Geometry check sheet. Reference: drawing and pictorial views, mm from the part's lowest x, y, z. A direction names the side the tool comes from. Give positions to 0.01 mm unless a question says otherwise; leave off trailing zeros. Write each loop counter-clockwise with the first axis right and the second up, starting at its lowest first coordinate (ties: lowest second). Pieces come first, ordered by that corner, then holes.
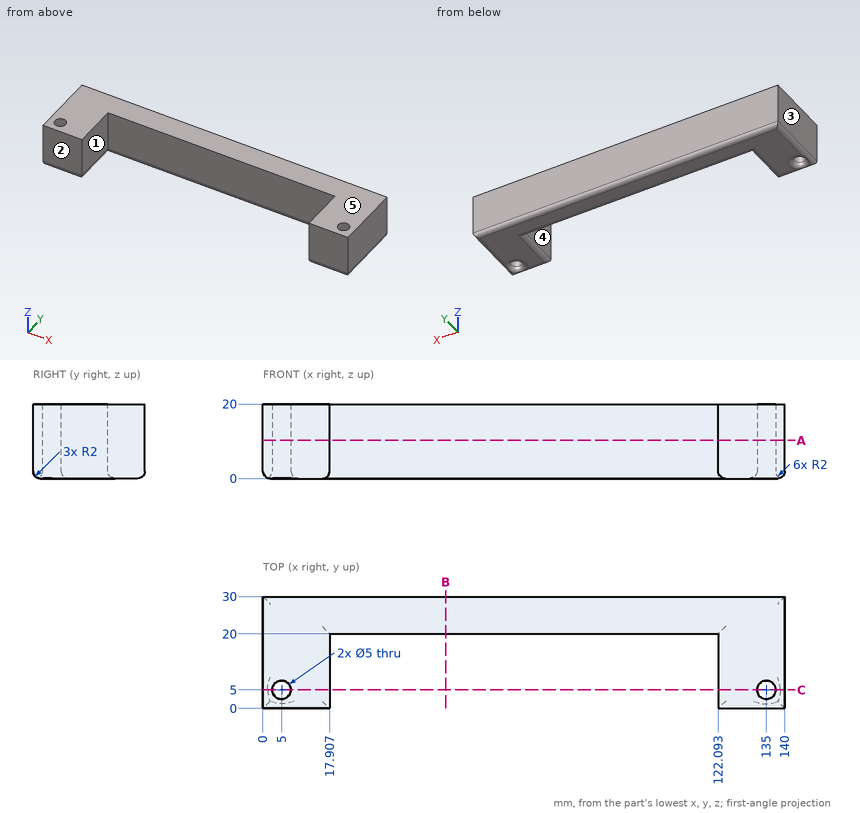
Item 1: Set-up check for the marked faces 1 and 2: record each of +Z, -Z, +X, -X, +Y, -Y from which the full face is reachable in a straight line by a thin tool's end or side.
Answer key:
face 1: +Z, -Z, -Y
face 2: +Z, -Z, +X, -X, -Y
Item 2: Depth check by flat-ended pin: pin 1 (6.5 mm diameter, centred on x = 5, y = 5, fed in from -Z); pin 2 (1 mm diameter, centred on x = 71, z = 17, fed in from -Y). Enter the tip coordinate at first touch or a pass-through.
Answer key:
pin 1: stops at z = 0.44
pin 2: stops at y = 20
Item 3: Sectioned sample at A-A on z = 10.25. Record the cut outline in (x, y), then the cut area to 3 significant figures.
Answer key:
outline: (0, 0) - (17.91, 0) - (17.91, 20) - (122.09, 20) - (122.09, 0) - (140, 0) - (140, 30) - (0, 30) - close; hole circle Ø5 at (5, 5); hole circle Ø5 at (135, 5)
area: 2,080 mm2
Item 4: Release check for a two-part mould opening along X. For the marked faces 3, 4 and 5 record: released by +X, released by -X, zero draft, split by the parting line, or undercut.
Answer key:
face 3: released by -X
face 4: undercut
face 5: zero draft
Item 5: Scan lines: line 1 along X through (y, z) = (19, 16.75); line 2 along Y through (x, z) = (5, 11.25); line 3 along X through (y, z) = (6, 12). Record each from-to range of solid material in increasing order.
Answer key:
line 1: x = 0 to 17.91, 122.09 to 140
line 2: y = 0 to 2.5, 7.5 to 30
line 3: x = 0 to 2.71, 7.29 to 17.91, 122.09 to 132.71, 137.29 to 140
Item 6: Sectioned sample at C-C on y = 5. State how many separate pieces and enclosed holes the cut face has, then the cut area to 3 significant figures.
Answer key:
separate pieces: 4
enclosed holes: 0
area: 510 mm2
Item 7: Sectioned sample at B-B on x = 49. Record the cut outline in (y, z).
Answer key:
outline: (20, 2) arc R2 ccw to (22, 0) - (28, 0) arc R2 ccw to (30, 2) - (30, 20) - (20, 20) - close
